Read the model definition and answer for the solid it produces. Units are mm, in the model's axes. Coordinates: 2 decimals unless noted, no trailing zeros. Loops run counter-clockwise (first coordinate to the right, second up) from the corner with the lowest first, then second, coordinate; pieces in that order, holes last.
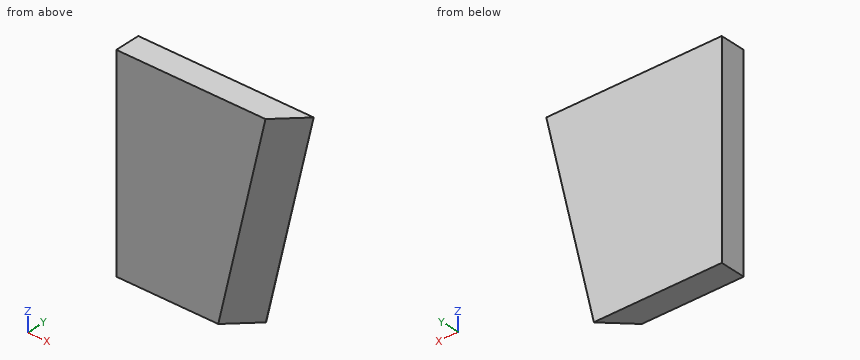
from build123d import *

# Parameters (mm, degrees)
F1_DEPTH = 12.7
F4_DEPTH = 118.595184


with BuildPart() as f1:
    # F0 (on Front) → F1 (new body)
    with BuildSketch(Plane.XZ):
        Polygon((87.122, 0), (0, 0), (0, -101.6), (63.5, -101.6), align=None)
    extrude(amount=F1_DEPTH)

    # F3 (on face) → F4 (cut, through all)
    with BuildSketch(Plane(origin=(4.408633, 0, 19.095886), x_dir=(0.97437, 0, -0.224951), z_dir=(-0.224951, 0, -0.97437))):
        Polygon((84.889069, 12.7), (72.189069, 12.7), (84.889069, 0), align=None)
    extrude(amount=F4_DEPTH, mode=Mode.SUBTRACT)


solid = f1.part
Q1. A cutting plane is placed at D-D (y = -11.5). Give the vertices of the cut face in (x, z), then the cut area to 3 significant figures.
Findings below:
outline: (0, -101.6) - (51.86, -101.6) - (75.32, 0) - (0, 0) - close
area: 6,460 mm2
Q2. A cutting plane is placed at A-A (z = -81.5). Give the vertices of the cut face in (x, y), then the cut area to 3 significant figures.
Findings below:
outline: (0, -12.7) - (55.27, -12.7) - (68.17, -0.13) - (68.17, 0) - (0, 0) - close
area: 785 mm2
Q3. A flat-ended cylindrical pin translates along its axis: pin 1 Ø8 at (x, z) = (63, -70.5) entering from -Y. Find the tip coordinate at first contact, or state that the pin passes through.
Findings below:
pin 1: stops at y = -11.64
Q4. A cutting plane is placed at C-C (x = 71.5). Give the vertices of the cut face in (y, z), then the cut area to 3 significant figures.
Findings below:
outline: (-12.7, -11.21) - (-0.11, -67.19) - (0, -67.19) - (0, 0) - (-12.7, 0) - close
area: 501 mm2
Q5. A cutting plane is placed at B-B (y = -5.25). Give the vertices of the cut face in (x, z).
Findings below:
outline: (0, -101.6) - (58.28, -101.6) - (81.73, 0) - (0, 0) - close
Q6. Straight lines are drawn through the part: probe 1 along Y at (x, z) = (63.5, -72.5); probe 2 along Y at (x, z) = (64, -94); probe 3 along X at (y, z) = (-9.75, -80). For each, find the intervals that lie inside material, in ascending order.
Findings below:
probe 1: y = -6.71 to 0
probe 2: y = -1.38 to 0
probe 3: x = 0 to 58.65
